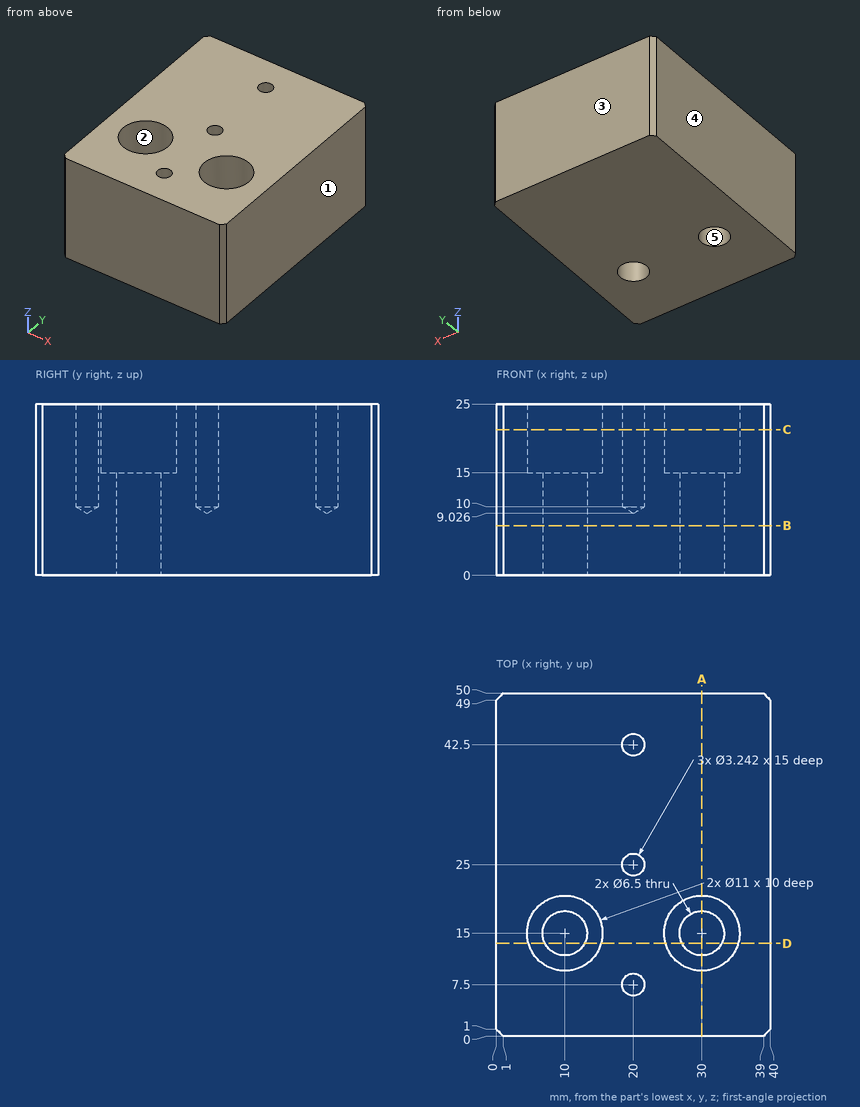
Geometry check sheet. Reference: drawing and pictorial views, mm from the part's lowest x, y, z. A direction names the side the tool comes from. Round coordinates to 2 decimals unless told otherwise and drop trailing zeros. Write each loop counter-clockwise with the first axis right and the second up, starting at its lowest first coordinate (ties: lowest second). Pieces come first, ordered by that corner, then holes.
(1) Section check A-A (x = 30). Enter the section's corners in (y, z), plus the area to 3 significant figures.
Returned:
outline: (0, 0) - (11.75, 0) - (11.75, 15) - (9.5, 15) - (9.5, 25) - (0, 25) - close; (18.25, 0) - (50, 0) - (50, 25) - (20.5, 25) - (20.5, 15) - (18.25, 15) - close
area: 1,040 mm2
(2) Access from +Z, -Z, +X, -X, +Y, -Y to the whole of each face (thin tool, end or side, straight path). Record for the marked faces 1 and 2.
Returned:
face 1: +Z, -Z, +X, +Y, -Y
face 2: +Z
(3) Mould release check, pull along X, two halves, no side actions. Record for the marked faces 3, 4 and 5: pulls with the +X half, pulls with the -X half, needs draft (parallel to the pull), parting line crosses it, or undercut.
Returned:
face 3: needs draft
face 4: pulls with the -X half
face 5: undercut
(4) Section check B-B (z = 7.25). Enter the section's corners in (x, y), plus the area to 3 significant figures.
Returned:
outline: (0, 1) - (1, 0) - (39, 0) - (40, 1) - (40, 49) - (39, 50) - (1, 50) - (0, 49) - close; hole circle Ø6.5 at (10, 15); hole circle Ø6.5 at (30, 15)
area: 1,930 mm2
(5) Material ranges on line 1 (X direction, y = 15, z = 21.5); line 2 (X direction, y = 15, z = 6.75); line 3 (X direction, y = 42.5, z = 15.5), recorded low to high.
Returned:
line 1: x = 0 to 4.5, 15.5 to 24.5, 35.5 to 40
line 2: x = 0 to 6.75, 13.25 to 26.75, 33.25 to 40
line 3: x = 0 to 18.38, 21.62 to 40
(6) Section check D-D (y = 13.5). Enter the section's corners in (x, z).
Returned:
outline: (0, 0) - (7.12, 0) - (7.12, 15) - (4.71, 15) - (4.71, 25) - (0, 25) - close; (12.88, 0) - (27.12, 0) - (27.12, 15) - (24.71, 15) - (24.71, 25) - (15.29, 25) - (15.29, 15) - (12.88, 15) - close; (32.88, 0) - (40, 0) - (40, 25) - (35.29, 25) - (35.29, 15) - (32.88, 15) - close
(7) Section check C-C (z = 21.25). Enter the section's corners in (x, y).
Returned:
outline: (0, 1) - (1, 0) - (39, 0) - (40, 1) - (40, 49) - (39, 50) - (1, 50) - (0, 49) - close; hole circle Ø11 at (10, 15); hole circle Ø3.24 at (20, 7.5); hole circle Ø3.24 at (20, 25); hole circle Ø3.24 at (20, 42.5); hole circle Ø11 at (30, 15)
